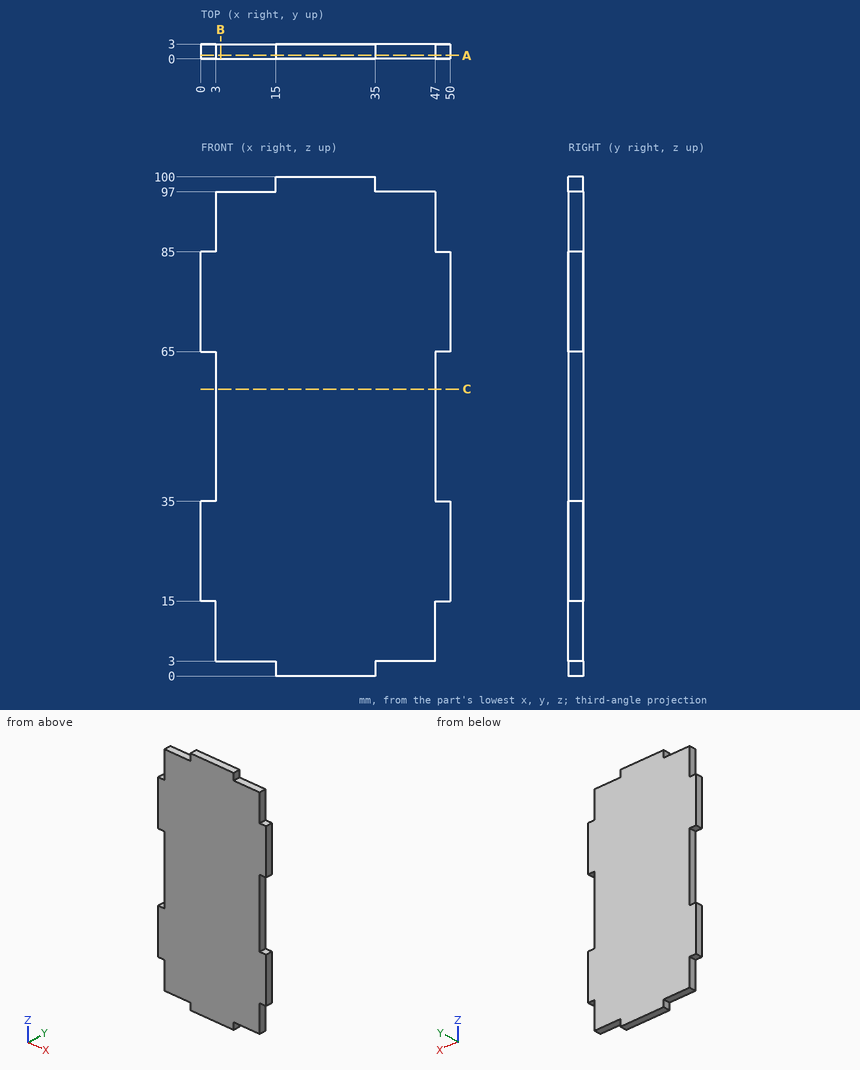
The drawing under review shows one solid part. Ordinate dimensions are in mm from its lowest x, y, z. Coordinates: 2 decimals unless noted, no trailing zeros. Order: outer loops, then holes, each group sorted by start corner. A loop starts at its lowest first (then second) coordinate and runs counter-clockwise, first axis right, second up. Notation, with made-up numbers: (-38, -6.5) -> (20, -6.5) arc R31 ccw to (20, 24.5) -> close; hole circle Ø6 at (-4, 87.25). An arc over 180 degrees is marked (long way). Return JSON: item names as keys, results as strings.
1. We need section A-A on y = 0.7. Write out the cut boundary in (x, z), and give its area (3 significant figures).
Answer block:
{"outline": "(0, 15) -> (3, 15) -> (3, 3) -> (15, 3) -> (15, 0) -> (35, 0) -> (35, 3) -> (47, 3) -> (47, 15) -> (50, 15) -> (50, 35) -> (47, 35) -> (47, 65) -> (50, 65) -> (50, 85) -> (47, 85) -> (47, 97) -> (35, 97) -> (35, 100) -> (15, 100) -> (15, 97) -> (3, 97) -> (3, 85) -> (0, 85) -> (0, 65) -> (3, 65) -> (3, 35) -> (0, 35) -> close", "area": "4,500 mm²"}
2. We need section B-B on x = 4. Write out the cut boundary in (y, z).
Answer block:
{"outline": "(0, 3) -> (3, 3) -> (3, 97) -> (0, 97) -> close"}
3. For pin 1 Ø0.9 at (y, z) = (1.5, 1.5) entering from +X; pin 2 Ø1.5 at (x, y) = (49, 1) entering from +Z; pin 3 Ø1.5 at (x, y) = (41, 1) entering from -Z, all flat-tipped, find the tip position at first contact; note any pin that passes through.
Answer block:
{"pin 1": "x = 35", "pin 2": "z = 85", "pin 3": "z = 3"}
4. For line 1 (X direction, y = 1.45, z = 59); line 2 (Z direction, x = 13, y = 0.65), list the stretches that pass through material, from the lowest coordinate up. Write a range as from..to.
Answer block:
{"line 1": "3..47", "line 2": "3..97"}
5. We need section C-C on z = 57.5. Write out the cut boundary in (x, y), and give its area (3 significant figures).
Answer block:
{"outline": "(3, 0) -> (47, 0) -> (47, 3) -> (3, 3) -> close", "area": "132 mm²"}
